from build123d import *

# Parameters (mm, degrees)
SKETCH_R        = 5
PAD_DEPTH       = 9
SKETCH005_R     = 2.2
POCKET_DEPTH    = 25.501
SKETCH006_R     = 8
POCKET001_DEPTH = 5.1
SKETCH007_R     = 4.125
POCKET002_DEPTH = 4.2
FILLET_R        = 3


with BuildPart() as filletbody:
    # Sketch → Pad (new body, symmetric)
    with BuildSketch(Plane.XY):
        with BuildLine():
            Line((-6, 25.5), (6, 25.5))
            ThreePointArc((12, 19.5), (10.242641, 23.742641), (6, 25.5))
            Line((12, 19.5), (12, 16))
            ThreePointArc((12, 16), (13.757359, 11.757359), (18, 10))
            Line((18, 10), (39, 10))
            Line((39, 10), (39, 0))
            Line((39, 0), (-27, 0))
            Line((-27, 0), (-27, 10))
            Line((-27, 10), (-20, 10))
            ThreePointArc((-20, 10), (-14.343146, 12.343146), (-12, 18))
            Line((-12, 18), (-12, 19.5))
            ThreePointArc((-6, 25.5), (-10.242641, 23.742641), (-12, 19.5))
        make_face()
        with Locations((0, 13.5)):
            Circle(SKETCH_R, mode=Mode.SUBTRACT)
    extrude(amount=PAD_DEPTH, both=True)

    # Sketch005 (on Face7 of Pad) → Pocket (cut, through all)
    with BuildSketch(Plane.XZ):
        with Locations((29, 0)):
            Circle(SKETCH005_R)
        with Locations((-18, 0)):
            Circle(SKETCH005_R)
    extrude(amount=-POCKET_DEPTH, mode=Mode.SUBTRACT)

    # Sketch006 (on Face5 of Pocket) → Pocket001 (cut)
    with BuildSketch(Plane.XY.offset(9)):
        with Locations((0, 13.5)):
            Circle(SKETCH006_R)
    extrude(amount=-POCKET001_DEPTH, mode=Mode.SUBTRACT)

    # Sketch007 (on Face9 of Pocket001) → Pocket002 (cut, symmetric)
    with BuildSketch(Plane(origin=(0, 10, 0), x_dir=(-1, 0, 0), z_dir=(0, 1, 0))):
        with Locations((18, 0)):
            Circle(SKETCH007_R)
        with Locations((-29, 0)):
            Circle(SKETCH007_R)
    extrude(amount=POCKET002_DEPTH, both=True, mode=Mode.SUBTRACT)

    # Fillet
    fillet_edges = [filletbody.edges().sort_by_distance(p)[0] for p in [
        (39, 10, 0),
        (-27, 10, 0),
    ]]
    fillet(fillet_edges, radius=FILLET_R)


with BuildPart() as part_mirroring:
    # Part__Mirroring: instance of FilletBody
    add(filletbody.part.mirror(Plane(origin=(0, 0, 0), x_dir=(0, -1, 0), z_dir=(1, 0, 0))))


solid = part_mirroring.part
Build history of the part. All positions in model axes, mm. A direction names the side the tool comes from. Round coordinates to 2 decimals unless told otherwise and drop trailing zeros. Loops run counter-clockwise (first coordinate to the right, second up) from the corner with the lowest first, then second, coordinate; pieces in that order, holes last. Notation, with made-up numbers: (32.25, 84) -> (60.25, 84) arc R25 ccw to (60.25, 105) -> close; hole circle Ø7 at (-33, -13). An arc over 180 degrees is marked (long way). Answer in a Markdown table with one row per item.
Item 1: Saw through at D-D (y = 13.5). Write the cut outline in (x, z).
Answers below:
| item | result |
|---|---|
| outline | (-12.55, -9) -> (-5, -9) -> (-5, 3.9) -> (-8, 3.9) -> (-8, 9) -> (-12.55, 9) -> close; (5, -9) -> (13.39, -9) -> (13.39, 9) -> (8, 9) -> (8, 3.9) -> (5, 3.9) -> close |
Item 2: Mould opens along Y. For faces 6 (the flat face through (-6, 7, 9)), 7 (the cylindrical face through (-7.63, 15.9, 6.49)), 8 (the flat face through (-6, 0, 0)) say: +Y half, -Y half, draft (parallel to the pull), parting line (faces both ways), or undercut.
Answers below:
| item | result |
|---|---|
| face 6 | draft |
| face 7 | undercut |
| face 8 | -Y half |
Item 3: Drill centre lines: L1, parallel to Z at x = -29, y = 3.8; L2, parallel to X at y = 6.75, z = 1.75; L3, parallel to Z at x = -29, y = 9 (3 decimals). Where is each one in solid material? Low to high. Write a range as [from, to].
Answers below:
| item | result |
|---|---|
| L1 | z = [-9, -2.2], [2.2, 9] |
| L2 | x = [-39, -32.74], [-25.26, 14.26], [21.74, 27] |
| L3 | z = [-9, -4.125], [4.125, 9] |
Item 4: Saw through at A-A (x = 0). Write the cut outline in (y, z), and give its area (3 significant figures).
Answers below:
| item | result |
|---|---|
| outline | (0, -9) -> (8.5, -9) -> (8.5, 3.9) -> (5.5, 3.9) -> (5.5, 9) -> (0, 9) -> close; (18.5, -9) -> (25.5, -9) -> (25.5, 9) -> (21.5, 9) -> (21.5, 3.9) -> (18.5, 3.9) -> close |
| area | 248 mm² |
Item 5: Saw through at C-C (z = 5.75). Write the cut outline in (x, y), and give its area (3 significant figures).
Answers below:
| item | result |
|---|---|
| outline | (-39, 0) -> (27, 0) -> (27, 7) arc R3 ccw to (24, 10) -> (20, 10) arc R8 cw to (12, 18) -> (12, 19.5) arc R6 ccw to (6, 25.5) -> (-6, 25.5) arc R6 ccw to (-12, 19.5) -> (-12, 16) arc R6 cw to (-18, 10) -> (-36, 10) arc R3 ccw to (-39, 7) -> close; hole circle Ø16 at (0, 13.5) |
| area | 833 mm² |
Item 6: Saw through at B-B (y = 9.25). Write the cut outline in (x, z) (3 decimals), and give its area (3 significant figures).
Answers below:
| item | result |
|---|---|
| outline | (-37.984, -9) -> (-2.634, -9) -> (-2.634, 3.9) -> (-6.778, 3.9) -> (-6.778, 9) -> (-37.984, 9) -> close; (2.634, -9) -> (25.984, -9) -> (25.984, 9) -> (6.778, 9) -> (6.778, 3.9) -> (2.634, 3.9) -> close; hole circle Ø8.25 at (-29, 0); hole circle Ø8.25 at (18, 0) |
| area | 907 mm² |
Item 7: Which spindle directions (+Z, -Z, +X, -X, +Y, -Y) get a long thin tool onto all of the face, cutting with end or side? Do faces 1 (the flat face through (12, 19, 0)), 2 (the flat face through (4, 10, 3.9)), 3 (the cylindrical face through (-33.12, 7.93, 0.18)), 4 (the flat face through (-39, 4, 0)), 5 (the flat face through (-25, 10, 2)). Say none if no direction does.
Answers below:
| item | result |
|---|---|
| face 1 | +Z, -Z, +X, +Y |
| face 2 | +Z |
| face 3 | +Y |
| face 4 | +Z, -Z, -X, +Y, -Y |
| face 5 | +Z, -Z, -X, +Y |
Item 8: Pin check, flat tips, straight feed: pin 1 (2 mm diameter, centred on x = 22, z = 2, fed in from +Y); pin 2 (0.8 mm diameter, centred on y = 18.5, z = -3, fed in from +X); pin 3 (1 mm diameter, centred on y = 18, z = 1.5, fed in from -X). Stop position of each tip, or through.
Answers below:
| item | result |
|---|---|
| pin 1 | stops at y = 10 |
| pin 2 | stops at x = 12 |
| pin 3 | stops at x = -12 |
